The listing builds one solid part. Answer for the finished solid, in the listing's coordinates (mm). Face numbers are marked on the shaded views. Coordinates: 2 decimals unless noted, no trailing zeros. Order: outer loops, then holes, each group sorted by start corner. A loop starts at its lowest first (then second) coordinate and runs counter-clockwise, first axis right, second up. Notation, with made-up numbers: (38.25, -22.75) -> (90.25, -22.75) arc R25 ccw to (90.25, 15.25) -> close; hole circle Ø9 at (22.5, 65). An arc over 180 degrees is marked (long way). Write item = value, one per line.
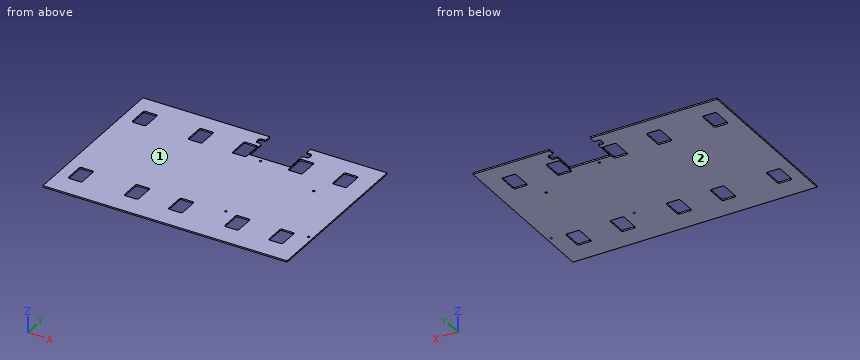
from build123d import *

# Parameters (mm, degrees)
SKETCH1_W           = 441.979400076
SKETCH1_H           = 305.81676
BOSS_EXTRUDE1_DEPTH = 2.54
CUT_EXTRUDE1_DEPTH  = 271.648139079
LPATTERN1_COUNT     = 3
LPATTERN1_PITCH     = 181.613999992
CUT_EXTRUDE2_DEPTH  = 271.648139079
LPATTERN2_COUNT     = 2
LPATTERN2_PITCH     = 181.613999992
CUT_EXTRUDE3_DEPTH  = 271.648139079
SKETCH6_R           = 2
CUT_EXTRUDE4_DEPTH  = 271.648139079


with BuildPart() as part:
    # Sketch1 → Boss-Extrude1 (new body)
    # profile 1 of 5: a face of its own
    with BuildSketch(Plane.XY):
        with Locations((0, -3.32067)):
            Rectangle(SKETCH1_W, SKETCH1_H)
        with BuildLine():
            ThreePointArc((-98.112625, -113.8), (-97.233945344, -115.921320344), (-95.112625, -116.8))
            Line((-95.112625, -116.8), (-75.712625, -116.8))
            ThreePointArc((-75.712625, -116.8), (-73.591304656, -115.921320344), (-72.712625, -113.8))
            Line((-72.712625, -113.8), (-72.712625, -81.7))
            ThreePointArc((-72.712625, -81.7), (-73.591304656, -79.578679656), (-75.712625, -78.7))
            Line((-75.712625, -78.7), (-95.112625, -78.7))
            ThreePointArc((-95.112625, -78.7), (-97.233945344, -79.578679656), (-98.112625, -81.7))
            Line((-98.112625, -81.7), (-98.112625, -113.8))
        make_face(mode=Mode.SUBTRACT)
        with BuildLine():
            ThreePointArc((-98.112625, 81.7), (-97.233945344, 79.578679656), (-95.112625, 78.7))
            Line((-95.112625, 78.7), (-75.712625, 78.7))
            ThreePointArc((-75.712625, 78.7), (-73.591304656, 79.578679656), (-72.712625, 81.7))
            Line((-72.712625, 81.7), (-72.712625, 113.8))
            ThreePointArc((-72.712625, 113.8), (-73.591304656, 115.921320344), (-75.712625, 116.8))
            Line((-75.712625, 116.8), (-95.112625, 116.8))
            ThreePointArc((-95.112625, 116.8), (-97.233945344, 115.921320344), (-98.112625, 113.8))
            Line((-98.112625, 113.8), (-98.112625, 81.7))
        make_face(mode=Mode.SUBTRACT)
        with BuildLine():
            ThreePointArc((-199.715375, -113.8), (-198.836695344, -115.921320344), (-196.715375, -116.8))
            Line((-196.715375, -116.8), (-177.315375, -116.8))
            ThreePointArc((-177.315375, -116.8), (-175.194054656, -115.921320344), (-174.315375, -113.8))
            Line((-174.315375, -113.8), (-174.315375, -81.7))
            ThreePointArc((-174.315375, -81.7), (-175.194054656, -79.578679656), (-177.315375, -78.7))
            Line((-177.315375, -78.7), (-196.715375, -78.7))
            ThreePointArc((-196.715375, -78.7), (-198.836695344, -79.578679656), (-199.715375, -81.7))
            Line((-199.715375, -81.7), (-199.715375, -113.8))
        make_face(mode=Mode.SUBTRACT)
        with BuildLine():
            ThreePointArc((-199.715375, 81.7), (-198.836695344, 79.578679656), (-196.715375, 78.7))
            Line((-196.715375, 78.7), (-177.315375, 78.7))
            ThreePointArc((-177.315375, 78.7), (-175.194054656, 79.578679656), (-174.315375, 81.7))
            Line((-174.315375, 81.7), (-174.315375, 113.8))
            ThreePointArc((-174.315375, 113.8), (-175.194054656, 115.921320344), (-177.315375, 116.8))
            Line((-177.315375, 116.8), (-196.715375, 116.8))
            ThreePointArc((-196.715375, 116.8), (-198.836695344, 115.921320344), (-199.715375, 113.8))
            Line((-199.715375, 113.8), (-199.715375, 81.7))
        make_face(mode=Mode.SUBTRACT)
    # profile 2 of 5: a face of its own
    with BuildSketch(Plane.XY):
        with BuildLine():
            Line((-199.715375, -113.8), (-199.715375, -81.7))
            ThreePointArc((-199.715375, -81.7), (-198.836695344, -79.578679656), (-196.715375, -78.7))
            Line((-196.715375, -78.7), (-177.315375, -78.7))
            ThreePointArc((-177.315375, -78.7), (-175.194054656, -79.578679656), (-174.315375, -81.7))
            Line((-174.315375, -81.7), (-174.315375, -113.8))
            ThreePointArc((-174.315375, -113.8), (-175.194054656, -115.921320344), (-177.315375, -116.8))
            Line((-177.315375, -116.8), (-196.715375, -116.8))
            ThreePointArc((-196.715375, -116.8), (-198.836695344, -115.921320344), (-199.715375, -113.8))
        make_face()
    # profile 3 of 5: a face of its own
    with BuildSketch(Plane.XY):
        with BuildLine():
            Line((-98.112625, -113.8), (-98.112625, -81.7))
            ThreePointArc((-98.112625, -81.7), (-97.233945344, -79.578679656), (-95.112625, -78.7))
            Line((-95.112625, -78.7), (-75.712625, -78.7))
            ThreePointArc((-75.712625, -78.7), (-73.591304656, -79.578679656), (-72.712625, -81.7))
            Line((-72.712625, -81.7), (-72.712625, -113.8))
            ThreePointArc((-72.712625, -113.8), (-73.591304656, -115.921320344), (-75.712625, -116.8))
            Line((-75.712625, -116.8), (-95.112625, -116.8))
            ThreePointArc((-95.112625, -116.8), (-97.233945344, -115.921320344), (-98.112625, -113.8))
        make_face()
    # profile 4 of 5: a face of its own
    with BuildSketch(Plane.XY):
        with BuildLine():
            Line((-199.715375, 113.8), (-199.715375, 81.7))
            ThreePointArc((-199.715375, 81.7), (-198.836695344, 79.578679656), (-196.715375, 78.7))
            Line((-196.715375, 78.7), (-177.315375, 78.7))
            ThreePointArc((-177.315375, 78.7), (-175.194054656, 79.578679656), (-174.315375, 81.7))
            Line((-174.315375, 81.7), (-174.315375, 113.8))
            ThreePointArc((-174.315375, 113.8), (-175.194054656, 115.921320344), (-177.315375, 116.8))
            Line((-177.315375, 116.8), (-196.715375, 116.8))
            ThreePointArc((-196.715375, 116.8), (-198.836695344, 115.921320344), (-199.715375, 113.8))
        make_face()
    # profile 5 of 5: a face of its own
    with BuildSketch(Plane.XY):
        with BuildLine():
            Line((-98.112625, 113.8), (-98.112625, 81.7))
            ThreePointArc((-98.112625, 81.7), (-97.233945344, 79.578679656), (-95.112625, 78.7))
            Line((-95.112625, 78.7), (-75.712625, 78.7))
            ThreePointArc((-75.712625, 78.7), (-73.591304656, 79.578679656), (-72.712625, 81.7))
            Line((-72.712625, 81.7), (-72.712625, 113.8))
            ThreePointArc((-72.712625, 113.8), (-73.591304656, 115.921320344), (-75.712625, 116.8))
            Line((-75.712625, 116.8), (-95.112625, 116.8))
            ThreePointArc((-95.112625, 116.8), (-97.233945344, 115.921320344), (-98.112625, 113.8))
        make_face()
    extrude(amount=BOSS_EXTRUDE1_DEPTH)

    # Sketch2 → Cut-Extrude1 (cut, through all)
    with BuildSketch(Plane.XY.offset(2.54)):
        with BuildLine():
            Line((-196.715375, 78.7), (-177.315375, 78.7))
            ThreePointArc((-177.315375, 78.7), (-175.194054656, 79.578679656), (-174.315375, 81.7))
            Line((-174.315375, 81.7), (-174.315375, 113.8))
            ThreePointArc((-174.315375, 113.8), (-175.194054656, 115.921320344), (-177.315375, 116.8))
            Line((-177.315375, 116.8), (-196.715375, 116.8))
            ThreePointArc((-196.715375, 116.8), (-198.836695344, 115.921320344), (-199.715375, 113.8))
            Line((-199.715375, 113.8), (-199.715375, 81.7))
            ThreePointArc((-199.715375, 81.7), (-198.836695344, 79.578679656), (-196.715375, 78.7))
        make_face()
        with BuildLine():
            Line((-199.715375, -81.7), (-199.715375, -113.8))
            ThreePointArc((-199.715375, -113.8), (-198.836695344, -115.921320344), (-196.715375, -116.8))
            Line((-196.715375, -116.8), (-177.315375, -116.8))
            ThreePointArc((-177.315375, -116.8), (-175.194054656, -115.921320344), (-174.315375, -113.8))
            Line((-174.315375, -113.8), (-174.315375, -81.7))
            ThreePointArc((-174.315375, -81.7), (-175.194054656, -79.578679656), (-177.315375, -78.7))
            Line((-177.315375, -78.7), (-196.715375, -78.7))
            ThreePointArc((-196.715375, -78.7), (-198.836695344, -79.578679656), (-199.715375, -81.7))
        make_face()
    cut_extrude1 = extrude(amount=-CUT_EXTRUDE1_DEPTH, mode=Mode.SUBTRACT)

    # LPattern1: Cut-Extrude1 ×3
    with Locations(*[(i * LPATTERN1_PITCH, 0, 0) for i in range(1, LPATTERN1_COUNT)]):
        add(cut_extrude1, mode=Mode.SUBTRACT)

    # Sketch3 → Cut-Extrude2 (cut, through all)
    with BuildSketch(Plane.XY.offset(2.54)):
        with BuildLine():
            Line((-72.712625, 81.7), (-72.712625, 113.8))
            ThreePointArc((-72.712625, 113.8), (-73.591304656, 115.921320344), (-75.712625, 116.8))
            Line((-75.712625, 116.8), (-95.112625, 116.8))
            ThreePointArc((-95.112625, 116.8), (-97.233945344, 115.921320344), (-98.112625, 113.8))
            Line((-98.112625, 113.8), (-98.112625, 81.7))
            ThreePointArc((-98.112625, 81.7), (-97.233945344, 79.578679656), (-95.112625, 78.7))
            Line((-95.112625, 78.7), (-75.712625, 78.7))
            ThreePointArc((-75.712625, 78.7), (-73.591304656, 79.578679656), (-72.712625, 81.7))
        make_face()
        with BuildLine():
            Line((-72.712625, -113.8), (-72.712625, -81.7))
            ThreePointArc((-72.712625, -81.7), (-73.591304656, -79.578679656), (-75.712625, -78.7))
            Line((-75.712625, -78.7), (-95.112625, -78.7))
            ThreePointArc((-95.112625, -78.7), (-97.233945344, -79.578679656), (-98.112625, -81.7))
            Line((-98.112625, -81.7), (-98.112625, -113.8))
            ThreePointArc((-98.112625, -113.8), (-97.233945344, -115.921320344), (-95.112625, -116.8))
            Line((-95.112625, -116.8), (-75.712625, -116.8))
            ThreePointArc((-75.712625, -116.8), (-73.591304656, -115.921320344), (-72.712625, -113.8))
        make_face()
    cut_extrude2 = extrude(amount=-CUT_EXTRUDE2_DEPTH, mode=Mode.SUBTRACT)

    # LPattern2: Cut-Extrude2 ×2
    with Locations(*[(i * LPATTERN2_PITCH, 0, 0) for i in range(1, LPATTERN2_COUNT)]):
        add(cut_extrude2, mode=Mode.SUBTRACT)

    # Sketch5 → Cut-Extrude3 (cut, through all)
    with BuildSketch(Plane.XY.offset(2.54)):
        with BuildLine():
            ThreePointArc((8.383999992, 139.78771), (7.802899846, 138.384810146), (6.399999992, 137.80371))
            Line((6.399999992, 137.80371), (1.399999992, 137.80371))
            ThreePointArc((1.399999992, 137.80371), (-1.439740841, 136.627450833), (-2.616000008, 133.78771))
            Line((-2.616000008, 133.78771), (-2.616000008, 128.78771))
            ThreePointArc((-2.616000008, 128.78771), (-1.439740841, 125.947969167), (1.399999992, 124.77171))
            Line((1.399999992, 124.77171), (6.399999992, 124.77171))
            ThreePointArc((6.399999992, 124.77171), (7.802899846, 124.190609854), (8.383999992, 122.78771))
            Line((8.383999992, 122.78771), (8.383999992, 87.77171))
            Line((8.383999992, 87.77171), (82.415999992, 87.77171))
            Line((82.415999992, 87.77171), (82.415999992, 122.78771))
            ThreePointArc((82.415999992, 122.78771), (82.997100138, 124.190609854), (84.399999992, 124.77171))
            Line((84.399999992, 124.77171), (89.399999992, 124.77171))
            ThreePointArc((89.399999992, 124.77171), (92.239740825, 125.947969167), (93.415999992, 128.78771))
            Line((93.415999992, 128.78771), (93.415999992, 133.78771))
            ThreePointArc((93.415999992, 133.78771), (92.239740825, 136.627450833), (89.399999992, 137.80371))
            Line((89.399999992, 137.80371), (84.399999992, 137.80371))
            ThreePointArc((84.399999992, 137.80371), (82.997100138, 138.384810146), (82.415999992, 139.78771))
            Line((82.415999992, 139.78771), (82.415999992, 149.80371))
            Line((82.415999992, 149.80371), (8.383999992, 149.80371))
            Line((8.383999992, 149.80371), (8.383999992, 139.78771))
        make_face()
    extrude(amount=-CUT_EXTRUDE3_DEPTH, mode=Mode.SUBTRACT)

    # Sketch6 → Cut-Extrude4 (cut, through all)
    with BuildSketch(Plane.XY.offset(2.54)):
        with Locations((63.425, -77.41229)):
            Circle(SKETCH6_R)
        with Locations((213.425, -77.41229)):
            Circle(SKETCH6_R)
        with Locations((150.425, 44.58771)):
            Circle(SKETCH6_R)
        with Locations((33.425, 79.58771)):
            Circle(SKETCH6_R)
    extrude(amount=-CUT_EXTRUDE4_DEPTH, mode=Mode.SUBTRACT)


solid = part.part
Q1. Find the intervals of material crossed by line 1 along X through (y, z) = (-114, 0.7); line 2 along Y through (x, z) = (-9, 0.25); line 3 along Y through (x, z) = (87, 0.2), in increasing order.
The answers:
line_1 = -220.99 to -199.71, -174.32 to -98.11, -72.72 to -18.09, 7.29 to 83.51, 108.89 to 163.52, 188.91 to 220.99
line_2 = -156.23 to -116.8, -78.7 to 78.7, 116.8 to 149.59
line_3 = -156.23 to -116.8, -78.7 to 78.7, 116.8 to 124.77, 137.8 to 149.59
Q2. The mould has two halves that part along Z. Classify the marked faces 1 and 2: released by +Z, released by -Z, zero draft, split by the parting line, or undercut.
The answers:
face_1 = released by +Z
face_2 = released by -Z
Q3. Section C-C, the plane x = 48 is taken. Give the vertices of the cut face in (y, z), plus the area to 3 significant figures.
The answers:
outline = (-156.23, 0) -> (87.77, 0) -> (87.77, 2.54) -> (-156.23, 2.54) -> close
area = 620 mm2
Q4. Section A-A, the plane x = -87 is taken. Give the vertices of the cut face in (y, z).
The answers:
outline = (-156.23, 0) -> (-116.8, 0) -> (-116.8, 2.54) -> (-156.23, 2.54) -> close; (-78.7, 0) -> (78.7, 0) -> (78.7, 2.54) -> (-78.7, 2.54) -> close; (116.8, 0) -> (149.59, 0) -> (149.59, 2.54) -> (116.8, 2.54) -> close
Q5. Section D-D, the plane z = 1.1 is taken. Give the number of separate pieces and of enclosed holes in the cut face, plus the area to 3 significant figures.
The answers:
separate_pieces = 1
enclosed_holes = 14
area = 121,000 mm2
Q6. Section B-B, the plane y = -105.5 is taken. Give the vertices of the cut face in (x, z), plus the area to 3 significant figures.
The answers:
outline = (-220.99, 0) -> (-199.72, 0) -> (-199.72, 2.54) -> (-220.99, 2.54) -> close; (-174.32, 0) -> (-98.11, 0) -> (-98.11, 2.54) -> (-174.32, 2.54) -> close; (-72.71, 0) -> (-18.1, 0) -> (-18.1, 2.54) -> (-72.71, 2.54) -> close; (7.3, 0) -> (83.5, 0) -> (83.5, 2.54) -> (7.3, 2.54) -> close; (108.9, 0) -> (163.51, 0) -> (163.51, 2.54) -> (108.9, 2.54) -> close; (188.91, 0) -> (220.99, 0) -> (220.99, 2.54) -> (188.91, 2.54) -> close
area = 800 mm2
